```python
from build123d import *

# Parameters (mm, degrees)
F1_DEPTH = 190.5
F2_R     = 6.35
F3_DEPTH = 21.9964
F4_R     = 3.175
F5_DEPTH = 103.867754064
F6_R     = 6.35
F7_DEPTH = 10.9982


with BuildPart() as f1:
    # F0 (on Front) → F1 (new body)
    with BuildSketch(Plane.XZ):
        with BuildLine():
            Line((8.139213971, 0), (-50.6065376103, 0))
            Line((-50.6065376103, 0), (-50.6065376103, -12.7))
            Line((-50.6065376103, -12.7), (20.2340623897, -12.7))
            Line((20.2340623897, -12.7), (125.5043623897, 169.633508128))
            Line((125.5043623897, 169.633508128), (114.5058397616, 175.983508128))
            Line((114.5058397616, 175.983508128), (15.282963971, 4.1244459855))
            ThreePointArc((15.282963971, 4.1244459855), (15.282963971, -4.1244459855), (8.139213971, 0))
        make_face()
    extrude(amount=F1_DEPTH)

    # F2 (on face) → F3 (join)
    with BuildSketch(Plane.XY):
        with Locations((-23.4285376103, -12.7)):
            Circle(F2_R)
    extrude(amount=F3_DEPTH)

    # F4 (on face) → F5 (cut, through all)
    with BuildSketch(Plane(origin=(9.6762854782, 0, -5.5866060256), x_dir=(0, -1, 0), z_dir=(-0.8660254038, 0, 0.5))):
        with Locations((152.4, 113.4483569855)):
            Circle(F4_R)
        with Locations((76.2, 113.4483569855)):
            Circle(F4_R)
        with Locations((12.7, 113.4483569855)):
            Circle(F4_R)
        with Locations((12.7, 164.2483569855)):
            Circle(F4_R)
    extrude(amount=-F5_DEPTH, mode=Mode.SUBTRACT)

    # F6 (on face) → F7 (join)
    with BuildSketch(Plane(origin=(9.6762854782, 0, -5.5866060256), x_dir=(0, -1, 0), z_dir=(-0.8660254038, 0, 0.5))):
        with Locations((12.7, 46.7733569855)):
            Circle(F6_R)
    extrude(amount=F7_DEPTH)


solid = f1.part
```
Here's how the part is built. I have some questions about the finished solid (model axes, mm). A direction names the side the tool comes from. Give positions to 0.01 mm unless a question says otherwise; leave off trailing zeros. Order: outer loops, then holes, each group sorted by start corner. A loop starts at its lowest first (then second) coordinate and runs counter-clockwise, first axis right, second up. Notation, with made-up numbers: (39, 24.5) -> (53, 24.5) arc R13 ccw to (53, 35.5) -> close; hole circle Ø10 at (30.25, -21). An arc over 180 degrees is marked (long way). Use CSV: the item, a comma, the result in double quotes. Start each with the question number.
Item 1: Suppose I cut it at B-B (y = -12.7). List the corners of the cut face in (x, z) for me (1 decimal).
Item 2: Suppose I cut it at D-D (z = 69). List the corners of the cut face in (x, y) for me.
Item 3: If I drill on probe 1 along Y at (x, z) = (-24, 13.5); probe 2 along Z at (x, y) = (12.5, -98.5); probe 3 along Z at (x, y) = (-41.5, -75), over which ranges is the centre line in solid material (lowest first)? Write a range as [from, to].
Item 4: Suppose I cut it at C-C (x = -37). List the corners of the cut face in (y, z) for me, and give its area (3 significant figures).
Item 5: Suppose I cut it at A-A (y = -57). List the corners of the cut face in (x, z) for me (1 decimal).
Item 6: On a 3-axis mill with a long thin cutter (end or side, diameter ignored), from which of +Z, -Z, +X, -X, +Y, -Y can I reach the whole of each face in a straight line? I mean faces 5 (the flat face through (-24, -13, 21.996)), 6 (the cylindrical face through (15.403, -93.916, -4.053)). Say none if no direction works.
Item 7: Thinking about a two-plate mould opening in Y: for faces 1 (the cylindrical face through (70.27, -12.01, 86.85)), 2 (the flat face through (50, -190.5, 61)), 3 (the cylindrical face through (-17.56, -15.13, 10.84)), 4 (the cylindrical face through (70.414, -77.665, 87.093)), which applies, pulls with the +Y half, pulls with the -Y half, needs draft (parallel to the pull), parting line crosses it, or undercut?
Item 8: I'm going to push flat-ended pins straight in: P1, Ø1, axis at x = 87, y = -152, coming from the +Z side; P2, Ø5, axis at x = 89.5, y = -156.5, coming from the +Z side; P3, Ø6.5, axis at x = -22, y = -14.5, coming from the +Z side. Where does each tip first touch, or does it pass through?
Answer block:
1,outline,"(-50.6, -12.7) -> (20.2, -12.7) -> (75.8, 83.6) -> (64.8, 89.9) -> (36.2, 40.4) -> (26.7, 45.9) -> (20.4, 34.9) -> (29.9, 29.4) -> (15.3, 4.1) arc R4.8 cw (long way) to (8.1, 0) -> (-17.1, 0) -> (-17.1, 22) -> (-29.8, 22) -> (-29.8, 0) -> (-50.6, 0) -> close; (68, 95.4) -> (79, 89.1) -> (101.2, 127.6) -> (90.2, 133.9) -> close; (93.4, 139.4) -> (104.4, 133.1) -> (125.5, 169.6) -> (114.5, 176) -> close"
2,outline,"(52.74, -190.5) -> (67.4, -190.5) -> (67.4, 0) -> (52.74, 0) -> close"
3,probe 1,"y = [-19.02, -6.38]"
3,probe 2,"z = [-12.7, -4.75]"
3,probe 3,"z = [-12.7, 0]"
4,outline,"(-190.5, -12.7) -> (0, -12.7) -> (0, 0) -> (-190.5, 0) -> close"
4,area,"2,420 mm^2"
5,outline,"(-50.6, -12.7) -> (20.2, -12.7) -> (125.5, 169.6) -> (114.5, 176) -> (15.3, 4.1) arc R4.8 cw (long way) to (8.1, 0) -> (-50.6, 0) -> close"
6,face 5,"+Z, -X, +Y, -Y"
6,face 6,"+Y, -Y"
7,face 1,"undercut"
7,face 2,"pulls with the -Y half"
7,face 3,"parting line crosses it"
7,face 4,"undercut"
8,P1,"stops at z = 129.21"
8,P2,"stops at z = 137"
8,P3,"stops at z = 22"
